from build123d import *

# Parameters (mm, degrees)
F1_DEPTH = 44.45
F2_DEPTH = 3.81
F3_DEPTH = 38.1
F5_DEPTH = 8.1202849069


with BuildPart() as f1:
    # F0 (on Front) → F1 (new body)
    with BuildSketch(Plane.XZ):
        with BuildLine():
            Line((23.84425, -8.7528133727), (25.4, 0))
            ThreePointArc((25.4, 0), (16.9476626833, 3.2174213406), (8.1062559696, 5.1209269282))
            ThreePointArc((8.1062559696, 5.1209269282), (0, 5.6739273919), (-8.1062559696, 5.1209269282))
            ThreePointArc((-8.1062559696, 5.1209269282), (-16.9476626833, 3.2174213406), (-25.4, 0))
            Line((-25.4, 0), (-23.84425, -8.7528133727))
            ThreePointArc((-23.84425, -8.7528133727), (-14.1597566071, -5.4872651146), (-4.0601424534, -3.9216944037))
            ThreePointArc((-4.0601424534, -3.9216944037), (0, -3.7834478897), (4.0601424534, -3.9216944037))
            ThreePointArc((4.0601424534, -3.9216944037), (14.1597566071, -5.4872651146), (23.84425, -8.7528133727))
        make_face()
    extrude(amount=F1_DEPTH)

    # F0 (on Front) → F2 (join)
    with BuildSketch(Plane.XZ):
        with BuildLine():
            ThreePointArc((-8.1062559696, 5.1209269282), (0, 5.6739273919), (8.1062559696, 5.1209269282))
            Line((8.1062559696, 5.1209269282), (8.1062559696, 17.8209269282))
            ThreePointArc((8.1062559696, 17.8209269282), (0, 25.9271828978), (-8.1062559696, 17.8209269282))
            Line((-8.1062559696, 17.8209269282), (-8.1062559696, 5.1209269282))
        make_face()
    extrude(amount=F2_DEPTH)

    # F0 (on Front) → F3 (join)
    with BuildSketch(Plane.XZ):
        with BuildLine():
            Line((4.0601424534, -25.0733971224), (4.0601424534, -3.9216944037))
            ThreePointArc((4.0601424534, -3.9216944037), (0, -3.7834478897), (-4.0601424534, -3.9216944037))
            Line((-4.0601424534, -3.9216944037), (-4.0601424534, -25.0733971224))
            Line((-4.0601424534, -25.0733971224), (0, -25.0733971224))
            Line((0, -25.0733971224), (4.0601424534, -25.0733971224))
        make_face()
    extrude(amount=F3_DEPTH)

    # F4 (on face) → F5 (cut, through all)
    with BuildSketch(Plane(origin=(-4.0601424534, 0, 0), x_dir=(0, -1, 0), z_dir=(-1, 0, 0))):
        Polygon((33.02, -3.9216944037), (5.08, -3.9216944037), (5.08, -21.8192890118), align=None)
        Polygon((38.1, -3.9216944037), (5.08, -25.0733971224), (38.1, -25.0733971224), align=None)
    extrude(amount=-F5_DEPTH, mode=Mode.SUBTRACT)


solid = f1.part
Check sheet for the modelled part. Datum: model origin and axes. Units: mm. A direction names the side the tool comes from. Give positions to 0.01 mm unless a question says otherwise; leave off trailing zeros. Loops run counter-clockwise (first coordinate to the right, second up) from the corner with the lowest first, then second, coordinate; pieces in that order, holes last. Notation, with made-up numbers: M 36,-18 L 75,-18 A21 ccw 75,2 Z; hole C 1.25,-26 d8. An arc over 180 degrees is marked long. Return JSON: item names as keys, results as strings. Group by question number.
1. Cross-section at A-A on x = 0. Record the boundary of the cut face in (y, z).
2. Go/stop test with flat-tipped pins: pin 1 (4 mm diameter, centred on x = -0.5, z = -17, fed in from -Y); pin 2 (6.5 mm diameter, centred on x = 1.5, y = -18.5, fed in from -Z); pin 3 (4 mm diameter, centred on y = -2.5, z = 14.5, fed in from +X); pin 4 (8 mm diameter, centred on x = -7.5, z = 14, fed in from +Y). Record where each tip stops, or that it passes through.
3. Thickness scan on L1, parallel to X at y = -2.5, z = -13; L2, parallel to Y at x = -5.5, z = 14.5; L3, parallel to Y at x = 4, z = -9. Record the ranges inside material, lowest first.
4. Cross-section at B-B on y = -11. Record the boundary of the cut face in (x, z).
5. Cross-section at D-D on z = -5. Record the boundary of the cut face in (x, y), plus the area to 3 significant figures.
6. Tool access check on faces 1 (the flat face through (4.06, -13, -17)), 2 (the flat face through (8.106, -2, 11)), 3 (the flat face through (-8.106, -2, 12)), 4 (the flat face through (-0.06, -18.85, -13)). Record the directions out of +Z, -Z, +X, -X, +Y, -Y that give a thin tool (end or side, any length) a straight path to the whole face; none if there is none.
7. Mould release check, pull along Y, two halves, no side actions. Record for faces 5 (the flat face through (24.61, -21.91, -4.44)), 6 (the flat face through (0, -19, -3.922)), 7 (the flat face through (0, -44.45, -1)): released by +Y, released by -Y, zero draft, split by the parting line, or undercut.
8. Cross-section at C-C on z = -20. Record the boundary of the cut face in (x, y), plus the area to 3 significant figures.
Return value:
{
 "1": {"outline": "M -44.45,-3.78 L -38.1,-3.78 L -38.1,-3.92 L -5.08,-25.07 L 0,-25.07 L 0,25.93 L -3.81,25.93 L -3.81,5.67 L -44.45,5.67 Z; hole M -33.02,-3.92 L -5.08,-21.82 L -5.08,-3.92 Z"},
 "2": {"pin 1": "y = -20.81", "pin 2": "z = -18.56", "pin 3": "x = 8.11", "pin 4": "y = 0"},
 "3": {"L1": "-4.06 to 4.06", "L2": "-3.81 to 0", "L3": "-30.17 to -25.09, -5.08 to 0"},
 "4": {"outline": "M -25.4,0 L -23.84,-8.75 A59.69 cw -4.06,-3.92 L 4.06,-3.92 A59.69 cw 23.84,-8.75 L 25.4,0 A59.69 ccw Z; M -4.06,-21.28 L 4.06,-21.28 L 4.06,-18.03 L -4.06,-18.03 Z"},
 "5": {"outline": "M -24.51,-44.45 L -11.99,-44.45 L -11.99,0 L -24.51,0 Z; M -4.06,-36.42 L 4.06,-36.42 L 4.06,-31.34 L -4.06,-31.34 Z; M -4.06,-5.08 L 4.06,-5.08 L 4.06,0 L -4.06,0 Z; M 11.99,-44.45 L 24.51,-44.45 L 24.51,0 L 11.99,0 Z", "area": "1,200 mm^2"},
 "6": {"face 1": "-Z, +Y, -Y", "face 2": "+Z, +X, +Y, -Y", "face 3": "+Z, -X, +Y, -Y", "face 4": "none"},
 "7": {"face 5": "zero draft", "face 6": "undercut", "face 7": "released by -Y"},
 "8": {"outline": "M -4.06,-13 L 4.06,-13 L 4.06,-7.92 L -4.06,-7.92 Z; M -4.06,-5.08 L 4.06,-5.08 L 4.06,0 L -4.06,0 Z", "area": "82.5 mm^2"}
}
